Part model, mm, in its own coordinate system. Face numbers are marked on the shaded views. A direction names the side the tool comes from. Coordinates: 2 decimals unless noted, no trailing zeros. Order: outer loops, then holes, each group sorted by start corner. A loop starts at its lowest first (then second) coordinate and runs counter-clockwise, first axis right, second up.
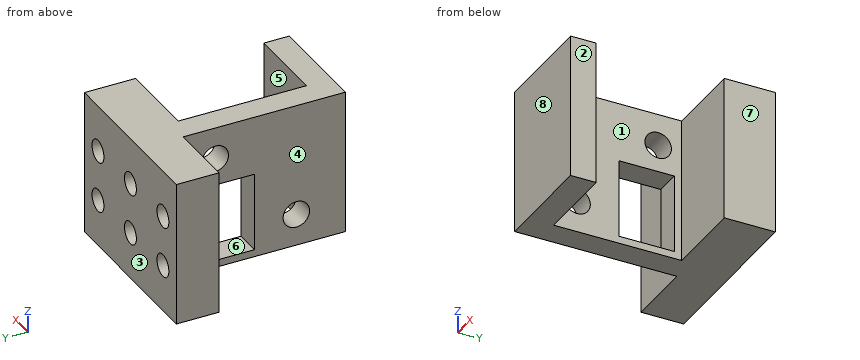
```python
from build123d import *

# Parameters (mm, degrees)
BOSS_EXTRUDE1_DEPTH           = 17
F_3_0_3_DIAMETER_HOLE1_D      = 3.1
TAP_DRILL_FOR_M2_5_TAP1_D     = 2.65
TAP_DRILL_FOR_M2_5_TAP1_DEPTH = 4.3
SKETCH8_W                     = 9.2
SKETCH8_H                     = 6.5
CUT_EXTRUDE1_DEPTH            = 10
SKETCH9_W                     = 8
SKETCH9_H                     = 6
BOSS_EXTRUDE2_DEPTH           = 17
TAP_DRILL_FOR_M2_5_TAP2_D     = 2.65
TAP_DRILL_FOR_M2_5_TAP2_DEPTH = 4.3
SKETCH12_W                    = 8
SKETCH12_H                    = 1
CUT_EXTRUDE2_DEPTH            = 26


with BuildPart() as part:
    # Sketch1 → Boss-Extrude1 (new body)
    with BuildSketch(Plane.XY):
        Polygon((0, 2.988929889), (0, 0), (5, 0), (12.5, 0), (12.5, 3), (3, 3), (3, 18), (12.5, 18), (12.5, 24), (5, 24), (0, 24), (0, 17.988929889), align=None)
    extrude(amount=BOSS_EXTRUDE1_DEPTH)

    # Ø3.0 (3) Diameter Hole1 (through all)
    with Locations(Plane(origin=(3, 0, 0), x_dir=(0, 0, -1), z_dir=(1, 0, 0))):
        with Locations((-13.25, 15.25), (-3.75, 5.75)):
            Hole(F_3_0_3_DIAMETER_HOLE1_D / 2)

    # Tap Drill for M2.5 Tap1
    with Locations(Plane(origin=(0, 24, 0), x_dir=(1, 0, 0), z_dir=(0, 1, 0))):
        with Locations((2.25, -5.5), (2.25, -11.5), (9.5, -11.5), (9.5, -5.5)):
            Hole(TAP_DRILL_FOR_M2_5_TAP1_D / 2, depth=TAP_DRILL_FOR_M2_5_TAP1_DEPTH)

    # Sketch8 → Cut-Extrude1 (cut)
    with BuildSketch(Plane(origin=(3, 0, 0), x_dir=(0, 0, -1), z_dir=(1, 0, 0))):
        with Locations((-5.45, 13.9)):
            Rectangle(SKETCH8_W, SKETCH8_H)
    extrude(amount=-CUT_EXTRUDE1_DEPTH, mode=Mode.SUBTRACT)

    # Sketch9 → Boss-Extrude2 (add)
    with BuildSketch(Plane.XY.offset(17)):
        with Locations((-4, 21)):
            Rectangle(SKETCH9_W, SKETCH9_H)
    extrude(amount=-BOSS_EXTRUDE2_DEPTH)

    # Tap Drill for M2.5 Tap2
    with Locations(Plane(origin=(0, 24, 0), x_dir=(1, 0, 0), z_dir=(0, 1, 0))):
        with Locations((-5, -11.5), (-5, -5.5)):
            Hole(TAP_DRILL_FOR_M2_5_TAP2_D / 2, depth=TAP_DRILL_FOR_M2_5_TAP2_DEPTH)

    # Sketch12 → Cut-Extrude2 (cut)
    with BuildSketch(Plane.XY.offset(17)):
        with Locations((-4, 18.5)):
            Rectangle(SKETCH12_W, SKETCH12_H)
    extrude(amount=-CUT_EXTRUDE2_DEPTH, mode=Mode.SUBTRACT)


solid = part.part
```
(1) Slice it at A-A, the plane y = 5.75. Give the cut face in (x, z).
(2) Drop flat-ended pins along their axis: pin 1 (3.5 mm diameter, centred on y = 15.25, z = 13.25, fed in from -X); pin 2 (0.8 mm diameter, centred on x = 9, z = 12, fed in from +Y); pin 3 (1.5 mm diameter, centred on x = -5.5, y = 18, fed in from -Z). Give the stop position or say it passes through.
(3) Slice it at D-D, the plane y = 15.25. Give the cut face in (x, z), then the cut area to 3 significant figures.
(4) Slice it at B-B, the plane x = 7.75. Give the cut face in (y, z).
(5) Tool access for the marked faces 4, 5, 6, 7 and 8: list every direction of +Z, -Z, +X, -X, +Y, -Y with a clear straight run to the whole face (end or side of a thin tool).
(6) Slice it at C-C, the plane z = 1.25. Give the cut face in (x, y), then the cut area to 3 significant figures.
(7) Pull direction Y, two halves, no side cores. Call the marked faces 1, 2 and 3: +Y half, -Y half, draft (parallel to the pull), parting line (faces both ways), or undercut.
(8) Probe line 1 (Z direction, x = -5, y = 21.6) (3 decimals); line 2 (Y direction, x = 2.25, z = 7); line 3 (Y direction, x = 5.75, z = 2). List the from-to ranges inside material, lowest first.
Here are the results:
1. outline: (0, 0) - (3, 0) - (3, 2.2) - (0, 2.2) - close; (0, 5.3) - (3, 5.3) - (3, 17) - (0, 17) - close
2. pin 1: stops at x = 0
2. pin 2: stops at y = 19.7
2. pin 3: passes through
3. outline: (0, 0) - (3, 0) - (3, 0.85) - (0, 0.85) - close; (0, 10.05) - (3, 10.05) - (3, 11.7) - (0, 11.7) - close; (0, 14.8) - (3, 14.8) - (3, 17) - (0, 17) - close
3. area: 14.1 mm2
4. outline: (0, 0) - (3, 0) - (3, 17) - (0, 17) - close; (18, 0) - (24, 0) - (24, 17) - (18, 17) - close
5. face 4: +Z, -Z, -X, -Y
5. face 5: +Z, -Z, +X
5. face 6: +X, -X
5. face 7: +Z, -Z, +X, +Y, -Y
5. face 8: +Z, -Z, +X, -X, -Y
6. outline: (-8, 19) - (0, 19) - (0, 17.15) - (3, 17.15) - (3, 18) - (12.5, 18) - (12.5, 24) - (-8, 24) - close; (0, 0) - (12.5, 0) - (12.5, 3) - (3, 3) - (3, 10.65) - (0, 10.65) - close
6. area: 178 mm2
7. face 1: undercut
7. face 2: draft
7. face 3: +Y half
8. line 1: z = 0 to 4.175, 6.825 to 10.175, 12.825 to 17
8. line 2: y = 0 to 10.65, 17.15 to 24
8. line 3: y = 0 to 3, 18 to 24
